Autodesk Inventor part; units mm, degrees
ref_plane "YZ Plane" through (0, 0, 0) normal (1, 0, 0) x (0, 1, 0)
ref_plane "XZ Plane" through (0, 0, 0) normal (0, 1, 0) x (-1, 0, 0)
ref_plane "XY Plane" through (0, 0, 0) normal (0, 0, 1) x (1, 0, 0)
sketch "Sketch1" plane through (0, 0, 0) normal (0, 0, 1) x (1, 0, 0)
  line L0 (16.5, 21.5) -> (16.5, 26.5)
  line L1 (16.5, 26.5) -> (16.5, 76.5)
  line L2 (16.5, 76.5) -> (26.5, 76.5)
  line L3 (26.5, 76.5) -> (26.5, 129.5)
  line L4 (26.5, 129.5) -> (-26.5, 129.5)
  line L5 (-26.5, 129.5) -> (-26.5, 76.5)
  line L6 (-26.5, 76.5) -> (-16.5, 76.5)
  line L7 (-16.5, 76.5) -> (-16.5, 26.5)
  line L8 (-16.5, 26.5) -> (-16.5, 21.5)
  line L9 (-16.5, 21.5) -> (-21.5, 21.5)
  line L10 (-21.5, 21.5) -> (-21.5, 11.5)
  line L11 (-21.5, 11.5) -> (-26.5, 11.5)
  line L12 (-26.5, 11.5) -> (-26.5, -11.5)
  line L13 (-26.5, -11.5) -> (-21.5, -11.5)
  line L14 (-21.5, -11.5) -> (-21.5, -21.5)
  line L15 (-21.5, -21.5) -> (-16.5, -21.5)
  line L16 (-16.5, -21.5) -> (-16.5, -26.5)
  line L17 (-16.5, -26.5) -> (-16.5, -76.5)
  line L18 (-16.5, -76.5) -> (-26.5, -76.5)
  line L19 (-26.5, -76.5) -> (-26.5, -129.5)
  line L20 (-26.5, -129.5) -> (26.5, -129.5)
  line L21 (26.5, -129.5) -> (26.5, -76.5)
  line L22 (26.5, -76.5) -> (16.5, -76.5)
  line L23 (16.5, -76.5) -> (16.5, -26.5)
  line L24 (16.5, -26.5) -> (16.5, -21.5)
  line L25 (16.5, -21.5) -> (21.5, -21.5)
  line L26 (21.5, -21.5) -> (21.5, -11.5)
  line L27 (21.5, -11.5) -> (26.5, -11.5)
  line L28 (26.5, -11.5) -> (26.5, 11.5)
  line L29 (26.5, 11.5) -> (21.5, 11.5)
  line L30 (21.5, 11.5) -> (21.5, 21.5)
  line L31 (21.5, 21.5) -> (16.5, 21.5)
  circle A0 centre (0, -103) radius 10.5
  circle A1 centre (0, 103) radius 10.5
  line L32 (-11.5, 26.5) -> (-11.5, 76.5)
  line L33 (-11.5, 76.5) -> (11.5, 76.5)
  line L34 (11.5, 76.5) -> (11.5, 26.5)
  line L35 (11.5, 26.5) -> (-11.5, 26.5)
  line L36 (11.5, -26.5) -> (11.5, -76.5)
  line L37 (11.5, -76.5) -> (-11.5, -76.5)
  line L38 (-11.5, -76.5) -> (-11.5, -26.5)
  line L39 (-11.5, -26.5) -> (11.5, -26.5)
  line L40 (-21, 21) -> (21, 21)
  line L41 (21, 21) -> (21, -21)
  line L42 (21, -21) -> (-21, -21)
  line L43 (-21, -21) -> (-21, 21)
  line L44 (-21, 21) -> (21, -21) construction
  line L45 (21, 21) -> (-21, -21) construction
  point P0 (0, 0)
  dimension "d0" = 42
  dimension "d1" = 42
extrude "Extrusion1" add sketch "Sketch1" along normal blind 33 contours L40 L41 L42 L43
sketch "Sketch2" plane through (0, 0, 33) normal (0, 0, 1) x (1, 0, 0)
  circle A0 centre (0, 0) radius 12.5
  dimension "d4" = 25
extrude "Extrusion2" add sketch "Sketch2" along normal blind 2
sketch "Sketch3" plane through (0, 0, 35) normal (0, 0, 1) x (1, 0, 0)
  circle A0 centre (0, 0) radius 2.5
  dimension "d7" = 5
extrude "Extrusion3" add sketch "Sketch3" along normal blind 20
properties part number "motor_sample"
Design review of the part built by this model. Coordinates are the model's own, in mm. A direction names the side the tool comes from. Coordinates: 2 decimals unless noted, no trailing zeros. Loops run counter-clockwise (first coordinate to the right, second up) from the corner with the lowest first, then second, coordinate; pieces in that order, holes last. Notation, with made-up numbers: M 10,49.25 L 20,49.25 A33 cw 20,78.25 Z; hole C -4,61.5 d6. An arc over 180 degrees is marked long. Answer as CSV lines item,"result".
Item 1: For probe 1 along Z at (x, y) = (8.5, 14); probe 2 along Z at (x, y) = (-4, 3), list the stretches that pass through material, from the lowest coordinate up.
Answer list:
probe 1,"0 to 33"
probe 2,"0 to 35"
Item 2: Add section A-A on y = 0. State the section outline as (x, z) points, plus the area to 3 significant figures.
Answer list:
outline,"M -21,0 L 21,0 L 21,33 L 12.5,33 L 12.5,35 L 2.5,35 L 2.5,55 L -2.5,55 L -2.5,35 L -12.5,35 L -12.5,33 L -21,33 Z"
area,"1,540 mm²"
Item 3: For P1, Ø4, axis at x = -9.5, y = -2.5, coming from the +Z side; P2, Ø2, axis at x = -3.5, z = 34.5, coming from the -Y side; P3, Ø1, axis at x = -9, y = -12.5, coming from the +Z side, all flat-tipped, find the tip position at first contact; note any pin that passes through.
Answer list:
P1,"z = 35"
P2,"y = -12.25"
P3,"z = 33"
Item 4: Add section C-C on x = 5. State the section outline as (y, z) points.
Answer list:
outline,"M -21,0 L 21,0 L 21,33 L 11.46,33 L 11.46,35 L -11.46,35 L -11.46,33 L -21,33 Z"
Item 5: Machinability: for faces 1 (the face through (-10, 10, 33)), 2 (the face through (0, 21, 16)), which of the approach directions +Z, -Z, +X, -X, +Y, -Y give a long, thin tool a straight path to every point of the face, cutting with its end or side? Answer none if there is none.
Answer list:
face 1,"+Z"
face 2,"+Z, -Z, +X, -X, +Y"
